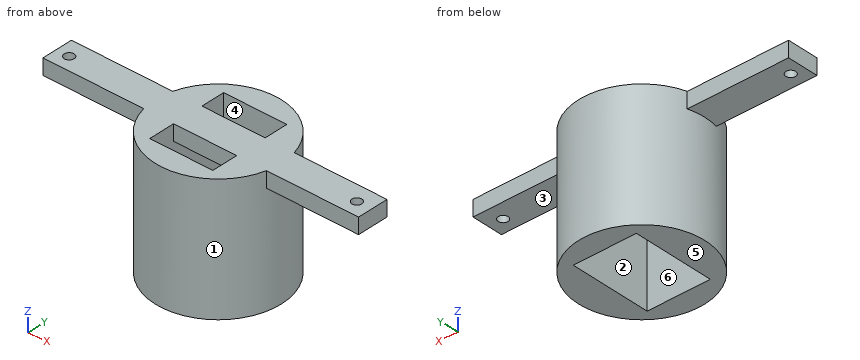
from build123d import *

# Parameters (mm, degrees)
F0_R      = 6.35
F1_DEPTH  = 12.7
F2_W      = 6.35
F2_H      = 8.255
F3_DEPTH  = 25.4
F4_W      = 31.75
F4_H      = 3.175
F5_DEPTH  = 1.5875
F6_R      = 0.4953
F7_DEPTH  = 1.5875
F9_R      = 0.4953
F10_DEPTH = 25.4


with BuildPart() as f1:
    # F0 (on Top) → F1 (new body)
    with BuildSketch(Plane.XY):
        Circle(F0_R)
    extrude(amount=F1_DEPTH)

    # F2 (on face) → F3 (cut)
    with BuildSketch(Plane.XY.offset(12.7)):
        Rectangle(F2_W, F2_H)
    extrude(amount=-F3_DEPTH, mode=Mode.SUBTRACT)

    # F4 (on face) → F5 (join)
    with BuildSketch(Plane.XY.offset(12.7)):
        with Locations((-0.4356827326, 0.1208083219)):
            Rectangle(F4_W, F4_H)
    extrude(amount=-F5_DEPTH)

    # F6 (on face) → F7 (cut)
    with BuildSketch(Plane.XY.offset(12.7)):
        with Locations((13.9489074385, 0)):
            Circle(F6_R)
    extrude(amount=-F7_DEPTH, mode=Mode.SUBTRACT)

    # F9 (on face) → F10 (cut)
    with BuildSketch(Plane.XY.offset(12.7)):
        with Locations((-14.99362, 0)):
            Circle(F9_R)
    extrude(amount=-F10_DEPTH, mode=Mode.SUBTRACT)


solid = f1.part
Input: part model. Units: mm. Frame: model coordinates. Face numbers are marked on the shaded views. A direction names the side the tool comes from. Coordinates: 2 decimals unless noted, no trailing zeros. Order: outer loops, then holes, each group sorted by start corner. A loop starts at its lowest first (then second) coordinate and runs counter-clockwise, first axis right, second up. Notation, with made-up numbers: M 38.25,-28 L 63.25,-28 A26 ccw 63.25,-14 Z; hole C 73,78 d10. An arc over 180 degrees is marked long. Answer in a Markdown table with one row per item.
(1) Section query A-A, the plane y = 0. Give the number of separate pieces and of enclosed holes in the cut face, plus the area to 3 significant figures.
Numbers:
| item | result |
|---|---|
| separate pieces | 3 |
| enclosed holes | 0 |
| area | 118 mm^2 |
(2) Contact query for flat-ended pins moving along their axis: pin 1 Ø6 at (x, z) = (-13, 9.5) entering from +Y; pin 2 Ø5 at (x, z) = (11, 10.5) entering from -Y; pin 3 Ø0.5 at (x, z) = (1, 12) entering from -Y. Output: stop coordinate, or through.
Numbers:
| item | result |
|---|---|
| pin 1 | stops at y = 1.71 |
| pin 2 | stops at y = -1.47 |
| pin 3 | stops at y = -6.31 |
(3) Material intervals for line 1 (X direction, y = -0.25, z = 9.5) (3 decimals); line 2 (X direction, y = -1.5, z = 3.25) (3 decimals); line 3 (Y direction, x = 5.5, z = 7.75), sorted ascending. Write a range as [from, to].
Numbers:
| item | result |
|---|---|
| line 1 | x = [-6.345, -3.175], [3.175, 6.345] |
| line 2 | x = [-6.17, -3.175], [3.175, 6.17] |
| line 3 | y = [-3.17, 3.17] |
(4) Section query C-C, the plane x = 0. Output: boundary loops of the cut face in (y, z), plus the area to 3 significant figures.
Numbers:
| item | result |
|---|---|
| outline | M -6.35,0 L -4.13,0 L -4.13,12.7 L -6.35,12.7 Z; M -1.47,11.11 L 1.71,11.11 L 1.71,12.7 L -1.47,12.7 Z; M 4.13,0 L 6.35,0 L 6.35,12.7 L 4.13,12.7 Z |
| area | 61.5 mm^2 |
(5) Section query D-D, the plane y = -2. Output: boundary loops of the cut face in (x, z) (3 decimals), plus the area to 3 significant figures.
Numbers:
| item | result |
|---|---|
| outline | M -6.027,0 L -3.175,0 L -3.175,12.7 L -6.027,12.7 Z; M 3.175,0 L 6.027,0 L 6.027,12.7 L 3.175,12.7 Z |
| area | 72.4 mm^2 |
(6) Draft query along X for the marked faces 1, 2, 3 and 4. Return one class per face: pulls with the +X half, pulls with the -X half, needs draft (parallel to the pull), parting line crosses it, or undercut.
Numbers:
| item | result |
|---|---|
| face 1 | parting line crosses it |
| face 2 | undercut |
| face 3 | needs draft |
| face 4 | undercut |
(7) Access query for the marked faces 5 and 6. Directions: +Z, -Z, +X, -X, +Y, -Y. A direction counts if a zero-diameter tool reaches every point of the face in a straight line with its end or side. Return the directions, or none.
Numbers:
| item | result |
|---|---|
| face 5 | -Z, +X, -X, +Y, -Y |
| face 6 | +Z, -Z |
